Can you work these out from the model? Positions are in its coordinate system, mm. A direction names the side the tool comes from. Give positions to 0.01 mm unless a question says otherwise; leave off trailing zeros. Write each loop counter-clockwise with the first axis right and the second up, starting at its lowest first coordinate (ties: lowest second). Pieces come first, ordered by that corner, then holes.
1. Suppose I cut it at B-B (x = 21). Please give me the cut outline in (y, z).
2. On a 3-axis mill with a long thin cutter (end or side, diameter ignored), from which of +Z, -Z, +X, -X, +Y, -Y can I reach the whole of each face in a straight line? I mean faces 4 (the flat face through (3, -34, 6)), 5 (the flat face through (0, -30, 6)). Say none if no direction works.
3. If I drill on probe 1 along Y at (x, z) = (21, 0.45); probe 2 along X at (y, z) = (-31, 7); probe 3 along Y at (x, z) = (30, 7.25), over which ranges is the centre line in solid material (lowest first)?
4. Suppose I cut it at D-D (y = -7). Please give me the cut outline in (x, z).
5. Suppose I cut it at A-A (y = -18). Please give me the cut outline in (x, z), and give its area (3 significant figures).
6. I'm going to push flat-ended pins straight in: pin 1 (3 mm diameter, centred on x = 10.5, y = -22.5, fed in from -Z); pin 2 (2 mm diameter, centred on x = 19, y = -11.5, fed in from +Z); pin 3 (5 mm diameter, centred on x = 30, z = 8.5, fed in from +Y). Where does each tip first touch, or does it pass through?
7. Suppose I cut it at C-C (z = 3.5). Please give me the cut outline in (x, y).
8. Thinking about a two-plate mould opening in X: for faces 1 (the flat face through (23, -15, 2)), 2 (the flat face through (46, -30, 6)), 3 (the flat face through (23, -40, 17)), which applies, pulls with the +X half, pulls with the -X half, needs draft (parallel to the pull), parting line crosses it, or undercut?
```python
from build123d import *

# Parameters (mm, degrees)
SKETCH1_W           = 46
SKETCH1_H           = 42
BOSS_EXTRUDE1_DEPTH = 2
SKETCH2_W           = 46
SKETCH2_H           = 3
BOSS_EXTRUDE2_DEPTH = 15
SKETCH4_R           = 5
CUT_EXTRUDE2_DEPTH  = 2
BOSS_EXTRUDE3_DEPTH = 3
BOSS_EXTRUDE4_DEPTH = 3


with BuildPart() as part:
    # Sketch1 → Boss-Extrude1 (new body)
    with BuildSketch(Plane.XY):
        with Locations((23, -21)):
            Rectangle(SKETCH1_W, SKETCH1_H)
    extrude(amount=BOSS_EXTRUDE1_DEPTH)

    # Sketch2 → Boss-Extrude2 (add)
    with BuildSketch(Plane.XY.offset(2)):
        with Locations((23, -40.5)):
            Rectangle(SKETCH2_W, SKETCH2_H)
    extrude(amount=BOSS_EXTRUDE2_DEPTH)

    # Sketch4 → Cut-Extrude2 (cut)
    with BuildSketch(Plane(origin=(0, 0, 0), x_dir=(-1, 0, 0), z_dir=(0, 0, -1))):
        with Locations((-21, -21)):
            Circle(SKETCH4_R)
    extrude(amount=-CUT_EXTRUDE2_DEPTH, mode=Mode.SUBTRACT)

    # Sketch5 → Boss-Extrude3 (add)
    with BuildSketch(Plane.ZY):
        Polygon((17, -39), (2, -21.123696111), (2, -39), align=None)
    extrude(amount=-BOSS_EXTRUDE3_DEPTH)

    # Sketch6 → Boss-Extrude4 (add)
    with BuildSketch(Plane(origin=(46, 0, 0), x_dir=(0, 0, -1), z_dir=(1, 0, 0))):
        Polygon((-17, -39), (-2, -21.123696111), (-2, -39), align=None)
    extrude(amount=-BOSS_EXTRUDE4_DEPTH)


solid = part.part
```
Checks:
1. outline: (-42, 0) - (-26, 0) - (-26, 2) - (-39, 2) - (-39, 17) - (-42, 17) - close; (-16, 0) - (0, 0) - (0, 2) - (-16, 2) - close
2. face 4: +Z, +Y
2. face 5: +Z, -Z, -X, +Y, -Y
3. probe 1: y = -42 to -26, -16 to 0
3. probe 2: x = 0 to 3, 43 to 46
3. probe 3: y = -42 to -39
4. outline: (0, 0) - (46, 0) - (46, 2) - (0, 2) - close
5. outline: (0, 0) - (17, 0) - (17, 2) - (0, 2) - close; (25, 0) - (46, 0) - (46, 2) - (25, 2) - close
5. area: 76.0 mm2
6. pin 1: stops at z = 0
6. pin 2: stops at z = 2
6. pin 3: stops at y = -39
7. outline: (0, -42) - (46, -42) - (46, -22.91) - (43, -22.91) - (43, -39) - (3, -39) - (3, -22.91) - (0, -22.91) - close
8. face 1: undercut
8. face 2: pulls with the +X half
8. face 3: needs draft
